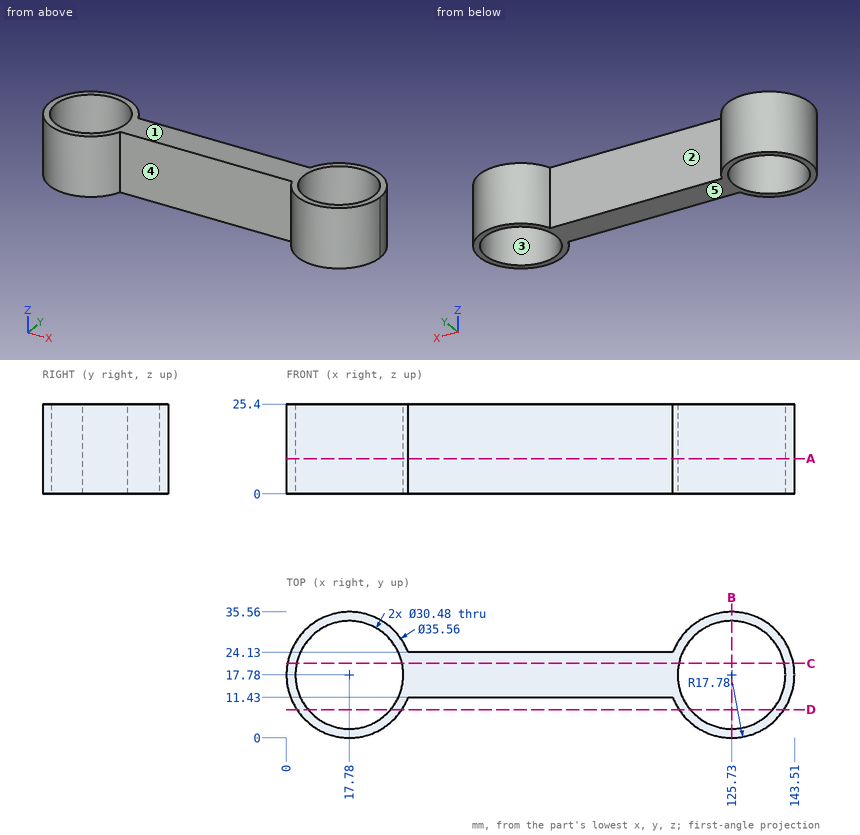
Input: dimensioned drawing with shaded views. Units: mm. Origin: part minimum x, y, z. A direction names the side the tool comes from. Coordinates: 2 decimals unless noted, no trailing zeros. Order: outer loops, then holes, each group sorted by start corner. A loop starts at its lowest first (then second) coordinate and runs counter-clockwise, first axis right, second up. Notation, with made-up numbers: (9, 44) -> (40, 44) arc R5 ccw to (40, 52) -> close; hole circle Ø11 at (-18, -9.75). An arc over 180 degrees is marked (long way). Answer in a Markdown table with one row per item.
Item 1: Ray query, L1, parallel to X at y = 18, z = 13.75; L2, parallel to Y at x = 125.73, z = 12; L3, parallel to X at y = 9, z = 22.75. Return the intervals inside material, ascending.
Return value:
| item | result |
|---|---|
| L1 | x = 0 to 2.54, 33.02 to 110.49, 140.97 to 143.51 |
| L2 | y = 0 to 2.54, 33.02 to 35.56 |
| L3 | x = 2.32 to 5.32, 30.24 to 33.24, 110.27 to 113.27, 138.19 to 141.19 |
Item 2: Section B-B on x = 125.73. Output: boundary loops of the cut face in (y, z).
Return value:
| item | result |
|---|---|
| outline | (0, 0) -> (2.54, 0) -> (2.54, 25.4) -> (0, 25.4) -> close; (33.02, 0) -> (35.56, 0) -> (35.56, 25.4) -> (33.02, 25.4) -> close |
Item 3: Section D-D on y = 8. Output: boundary loops of the cut face in (x, z).
Return value:
| item | result |
|---|---|
| outline | (2.93, 0) -> (6.09, 0) -> (6.09, 25.4) -> (2.93, 25.4) -> close; (29.47, 0) -> (32.63, 0) -> (32.63, 25.4) -> (29.47, 25.4) -> close; (110.88, 0) -> (114.04, 0) -> (114.04, 25.4) -> (110.88, 25.4) -> close; (137.42, 0) -> (140.58, 0) -> (140.58, 25.4) -> (137.42, 25.4) -> close |
Item 4: Access query for the marked faces 1 and 2. Directions: +Z, -Z, +X, -X, +Y, -Y. A direction counts if a zero-diameter tool reaches every point of the face in a straight line with its end or side. Return the directions, or none.
Return value:
| item | result |
|---|---|
| face 1 | +Z, +X, -X, +Y, -Y |
| face 2 | +Z, -Z, +Y |
Item 5: Section C-C on y = 21. Output: boundary loops of the cut face in (x, z).
Return value:
| item | result |
|---|---|
| outline | (0.29, 0) -> (2.88, 0) -> (2.88, 25.4) -> (0.29, 25.4) -> close; (32.68, 0) -> (110.83, 0) -> (110.83, 25.4) -> (32.68, 25.4) -> close; (140.63, 0) -> (143.22, 0) -> (143.22, 25.4) -> (140.63, 25.4) -> close |
Item 6: Draft query along X for the marked faces 3, 4 and 5. Return one class per face: released by +X, released by -X, zero draft, split by the parting line, or undercut.
Return value:
| item | result |
|---|---|
| face 3 | undercut |
| face 4 | undercut |
| face 5 | zero draft |
Item 7: Section A-A on z = 10. Output: boundary loops of the cut face in (x, y), plus the area to 3 significant figures.
Return value:
| item | result |
|---|---|
| outline | (34.39, 11.43) -> (109.12, 11.43) arc R17.78 ccw (long way) to (109.12, 24.13) -> (34.39, 24.13) arc R17.78 ccw (long way) to start; hole circle Ø30.48 at (17.78, 17.78); hole circle Ø30.48 at (125.73, 17.78) |
| area | 1,460 mm² |
Item 8: Contact query for flat-ended pins moving along their axis: P1, Ø7.5, axis at x = 85, z = 9.5, coming from the -Y side; P2, Ø12.5, axis at x = 75.5, z = 12.5, coming from the +Y side. Output: stop coordinate, or through.
Return value:
| item | result |
|---|---|
| P1 | stops at y = 11.43 |
| P2 | stops at y = 24.13 |
